```python
from build123d import *

# Parameters (mm, degrees)
SKETCH1_R           = 6.4999997
SKETCH1_R_2         = 1.999996
BOSS_EXTRUDE1_DEPTH = 4.99999


with BuildPart() as part:
    # Sketch1 → Boss-Extrude1 (new body)
    with BuildSketch(Plane.XY.offset(7)):
        with Locations(Location((0, 0, 0), (0, 0, 180))):
            Circle(SKETCH1_R)
        with Locations(Location((0, 0, 0), (0, 0, 180))):
            Circle(SKETCH1_R_2, mode=Mode.SUBTRACT)
    extrude(amount=-BOSS_EXTRUDE1_DEPTH)

    # Sketch4 → Cut-Revolve1 (revolve, cut)
    with BuildSketch(Plane(origin=(0, 0, 0), x_dir=(1, 0, 0), z_dir=(0, 1, 0)), mode=Mode.PRIVATE) as cut_revolve1_sk:
        Polygon((2.99999654, -2.4000092), (2.99999654, -2.00001), (5.49999916, -2.00001), (5.49999916, -2.4000092), (5.19999976, -2.4000092), (5.19999976, -2.202656618), (3.29999594, -2.202656618), (3.29999594, -2.4000092), align=None)
        Polygon((5.49999916, -7), (2.99999654, -7), (2.99999654, -6.6000008), (3.29999594, -6.6000008), (3.29999594, -6.797353382), (5.19999976, -6.797353382), (5.19999976, -6.6000008), (5.49999916, -6.6000008), align=None)
    revolve(cut_revolve1_sk.sketch.rotate(Axis((0, 0, 2.00001), (0, 0, 1)), 180), axis=Axis((0, 0, 2.00001), (0, 0, 1)), mode=Mode.SUBTRACT)


solid = part.part
```
The model under review builds one solid part; all positions refer to its coordinate system, in mm. A direction names the side the tool comes from. Round coordinates to 2 decimals unless told otherwise and drop trailing zeros. Loops run counter-clockwise (first coordinate to the right, second up) from the corner with the lowest first, then second, coordinate; pieces in that order, holes last.
1) Consider section C-C on y = 4. State the section outline as (x, z) points, then the cut area to 3 significant figures.
Values follow:
outline: (-5.12, 2) - (-3.77, 2) - (-3.77, 2.4) - (-3.32, 2.4) - (-3.32, 2.2) - (3.32, 2.2) - (3.32, 2.4) - (3.77, 2.4) - (3.77, 2) - (5.12, 2) - (5.12, 7) - (3.77, 7) - (3.77, 6.6) - (3.32, 6.6) - (3.32, 6.8) - (-3.32, 6.8) - (-3.32, 6.6) - (-3.77, 6.6) - (-3.77, 7) - (-5.12, 7) - close
area: 47.8 mm2
2) The part is to be moulded in two halves that separate along X. For faces 1 (the face through (-6.2, -1.95, 4.54)), 2 (the face through (-1, 2, 7)), 3 (the face through (3.4, 1.1, 6.797)), say which applies: pulls with the +X half, pulls with the -X half, needs draft (parallel to the pull), parting line crosses it, or undercut.
Values follow:
face 1: parting line crosses it
face 2: needs draft
face 3: undercut
3) Tool access review of faces 4 (the face through (5, -3, 2)), 5 (the face through (0.65, 2.93, 6.8)), 6 (the face through (0.65, 2.93, 2.2)): name each direction out of +Z, -Z, +X, -X, +Y, -Y from which nothing blocks a thin tool from reaching the whole face with its end or side.
Values follow:
face 4: -Z, +X, -X, +Y, -Y
face 5: +Z
face 6: -Z
4) Wall thickness on line 1 along Y through (x, z) = (0, 6.7); line 2 along Y through (x, z) = (0, 6.85); line 3 along Y through (x, z) = (0, 2.85): over which ranges is each line inside the solid? List them lowest first.
Values follow:
line 1: y = -6.5 to -5.5, -5.2 to -3.3, -3 to -2, 2 to 3, 3.3 to 5.2, 5.5 to 6.5
line 2: y = -6.5 to -5.5, -3 to -2, 2 to 3, 5.5 to 6.5
line 3: y = -6.5 to -2, 2 to 6.5
5) Consider section A-A on y = -5. State the section outline as (x, z) points, then the cut area to 3 significant figures.
Values follow:
outline: (-4.15, 2) - (-2.29, 2) - (-2.29, 2.4) - (-1.43, 2.4) - (-1.43, 2.2) - (1.43, 2.2) - (1.43, 2.4) - (2.29, 2.4) - (2.29, 2) - (4.15, 2) - (4.15, 7) - (2.29, 7) - (2.29, 6.6) - (1.43, 6.6) - (1.43, 6.8) - (-1.43, 6.8) - (-1.43, 6.6) - (-2.29, 6.6) - (-2.29, 7) - (-4.15, 7) - close
area: 39.0 mm2
6) Consider section B-B on z = 3.7. State the section outline as (x, y) points, then the cut area to 3 significant figures.
Values follow:
outline: circle Ø13 at (0, 0); hole circle Ø4 at (0, 0)
area: 120 mm2
